Autodesk Inventor part; units mm, degrees
ref_plane "YZ Plane" through (0, 0, 0) normal (1, 0, 0) x (0, 1, 0)
ref_plane "XZ Plane" through (0, 0, 0) normal (0, 1, 0) x (-1, 0, 0)
ref_plane "XY Plane" through (0, 0, 0) normal (0, 0, 1) x (1, 0, 0)
sketch "Sketch1" plane through (0, 0, 0) normal (0, 1, 0) x (-1, 0, 0)
  line L0 (0, 0) -> (0, -19.75)
  line L1 (0, -19.75) -> (-4.75, -19.75)
  line L2 (-4.75, -19.75) -> (-4.75, 0)
  line L3 (-4.75, 0) -> (0, 0)
  dimension "d0" = 19.75
  dimension "d1" = 4.75
extrude "Extrusion1" add sketch "Sketch1" along normal blind 15
sketch "Sketch3" plane through (0, 0, 0) normal (0, 0, 1) x (1, 0, 0)
  line L0 (0, 0) -> (0, -60)
  line L1 (4.75, 0) -> (0, 0)
  line L2 (0, 0) -> (0, -55)
  line L3 (0, 0) -> (0, -50)
  line L4 (0, 0) -> (35, 0)
  line L5 (4.75, 0) -> (39.75, 0)
  line L6 (0, 0) -> (35, -20)
  line L7 (4.75, 0) -> (39.75, -20)
  line L8 (35, -20) -> (39.75, -20)
  dimension "d4" = 60
  dimension "d5" = 55
  dimension "d6" = 50
  dimension "d7" = 35
  dimension "d8" = 35
  dimension "d23" = 20
  dimension "d24" = 20
extrude "Extrusion2" add sketch "Sketch3" against normal blind 19.75
sketch "Sketch4" plane through (35, -20, 0) normal (0, -1, 0) x (1, 0, 0)
  line L0 (0, 0) -> (0, -19.75)
  line L1 (0, -9.875) -> (0, 60.125)
  line L2 (0, -9.875) -> (0, -79.875)
  line L3 (0, -79.875) -> (40, -79.875)
  line L4 (40, -79.875) -> (40, 60.125)
  line L5 (40, 60.125) -> (0, 60.125)
  point P0 (-35, 0)
  dimension "d11" = 70
  dimension "d12" = 70
  dimension "d13" = 40
extrude "Extrusion3" add sketch "Sketch4" along normal blind 3
chamfer "Chamfer1" distance 1 angle 45 2 edges at (35, -21.5, 60.125) (35, -21.5, -79.875)
chamfer "Chamfer2" distance 7 angle 45 2 edges at (75, -21.5, 60.125) (75, -21.5, -79.875)
fillet "Fillet1" radius 2 4 edges at (75, -21.5, 53.125) (68, -21.5, 60.125) (75, -21.5, -72.875) (68, -21.5, -79.875)
properties part number "DudukanLineSensor"
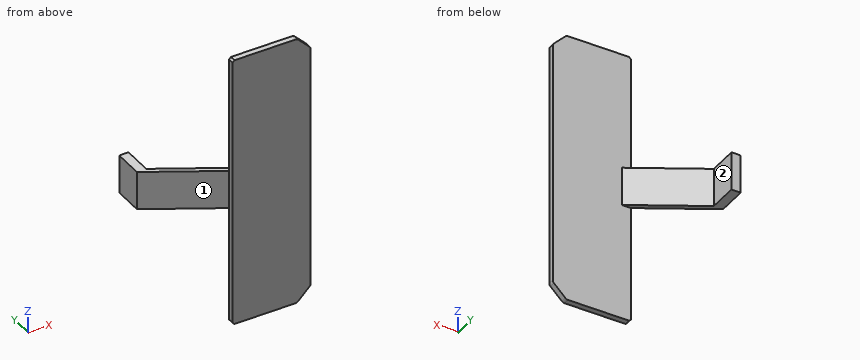
For this review, take the finished solid that the model builds, in its own axes (mm). Face numbers are marked on the shaded views. A direction names the side the tool comes from. Coordinates: 2 decimals unless noted, no trailing zeros. Write each loop counter-clockwise with the first axis right and the second up, starting at its lowest first coordinate (ties: lowest second). Pieces come first, ordered by that corner, then holes. Notation, with made-up numbers: (60.25, 81) - (67.25, 81) arc R6 cw to (67.25, 92) - close; hole circle Ø11 at (16, -38). An arc over 180 degrees is marked (long way). Put each result on its own line as item: value.
1. Add section A-A, the plane z = -5. Give the boundary of the cut face in (x, y), then the cut area to 3 significant figures.
Values found:
outline: (0, 0) - (35, -20) - (35, -23) - (75, -23) - (75, -20) - (39.75, -20) - (4.75, 0) - (4.75, 15) - (0, 15) - close
area: 286 mm²
2. Add section B-B, the plane x = 37.5. Give the boundary of the cut face in (y, z) (3 decimals).
Values found:
outline: (-23, -79.875) - (-20, -79.875) - (-20, -19.75) - (-18.714, -19.75) - (-18.714, 0) - (-20, 0) - (-20, 60.125) - (-23, 60.125) - close
3. Wall thickness on probe 1 along Z at (x, y) = (22.5, -11.5); probe 2 along Y at (x, z) = (43, 47); probe 3 along X at (y, z) = (-20.5, 5): over which ranges is each line inside the solid? List them lowest first.
Values found:
probe 1: -19.75 to 0
probe 2: -23 to -20
probe 3: 35 to 75
4. Machinability: for the marked faces 1 and 2, which of the approach directions +Z, -Z, +X, -X, +Y, -Y give a long, thin tool a straight path to every point of the face, cutting with its end or side? Answer none if there is none.
Values found:
face 1: +Z, -Z, -X, -Y
face 2: +Z, -Z, +X, +Y
5. For pin 1 (4 mm diameter, centred on x = 19, z = -12, fed in from -Y); pin 2 (5 mm diameter, centred on x = 19, z = 0, fed in from +Y); pin 3 (10 mm diameter, centred on y = 6, z = -23, fed in from +X); pin 4 (8 mm diameter, centred on x = 10, y = 10.5, fed in from +Z), all flat-tipped, find the tip position at first contact; note any pin that passes through.
Values found:
pin 1: y = -12
pin 2: y = -6.71
pin 3: x = 4.75
pin 4: through
6. Add section D-D, the plane x = 48. Give the boundary of the cut face in (y, z) (3 decimals), then the cut area to 3 significant figures.
Values found:
outline: (-23, -79.875) - (-20, -79.875) - (-20, 60.125) - (-23, 60.125) - close
area: 420 mm²
7. Add section C-C, the plane y = -10.5. Give the boundary of the cut face in (x, z) (3 decimals).
Values found:
outline: (18.375, -19.75) - (23.125, -19.75) - (23.125, 0) - (18.375, 0) - close
